Geometry check sheet. Reference: the model listing, model coordinates, mm. A direction names the side the tool comes from. Round coordinates to 2 decimals unless told otherwise and drop trailing zeros. Order: outer loops, then holes, each group sorted by start corner. A loop starts at its lowest first (then second) coordinate and runs counter-clockwise, first axis right, second up. Notation, with made-up numbers: M -23,10.5 L 32,10.5 A28 ccw 32,38.5 Z; hole C 26,-12 d6. An arc over 180 degrees is marked long. Answer as a JSON object with one key per item and string values. Group by question number.
```python
from build123d import *

# Parameters (mm, degrees)
F1_DEPTH = 12.7
F2_R     = 3.175
F3_DEPTH = 3.175
F4_R     = 3.175
F5_DEPTH = 3.175
F6_R     = 3.175
F7_DEPTH = 12.7


with BuildPart() as f1:
    # F0 (on Front) → F1 (new body)
    with BuildSketch(Plane.XZ):
        with BuildLine():
            Line((-8.975765, -6.223), (8.975765, -6.223))
            ThreePointArc((8.975765, -6.223), (0, 10.922), (-8.975765, -6.223))
        make_face()
    extrude(amount=F1_DEPTH)

    # F2 (on face) → F3 (join)
    with BuildSketch(Plane.XZ.offset(12.7)):
        Circle(F2_R)
    extrude(amount=F3_DEPTH)

    # F4 (on face) → F5 (join)
    with BuildSketch(Plane(origin=(0, 0, 0), x_dir=(-1, 0, 0), z_dir=(0, 1, 0))):
        Circle(F4_R)
    extrude(amount=F5_DEPTH)

    # F6 (on face) → F7 (cut)
    with BuildSketch(Plane(origin=(0, 0, -6.223), x_dir=(1, 0, 0), z_dir=(0, 0, -1))):
        with Locations((0, 6.35)):
            Circle(F6_R)
    extrude(amount=-F7_DEPTH, mode=Mode.SUBTRACT)


solid = f1.part
```
1) Sectioned sample at D-D (z = -4). Record the boundary of the cut face in (x, y) (3 decimals), then the cut area to 3 significant figures.
2) Sectioned sample at B-B (x = 0). Record the boundary of the cut face in (y, z) (3 decimals).
3) Sectioned sample at A-A (z = 0). Record the boundary of the cut face in (x, y) (3 decimals), then the cut area to 3 significant figures.
4) Set-up check for faces 1 (the flat face through (0, -6, 6.477)), 2 (the cylindrical face through (0.69, 1.57, -3.1)), 3 (the cylindrical face through (-0.69, -14.27, -3.1)): record each of +Z, -Z, +X, -X, +Y, -Y from which the full face is reachable in a straight line by a thin tool's end or side.
5) Sectioned sample at C-C (y = -6.35). Record the boundary of the cut face in (x, z) (3 decimals), then the cut area to 3 significant figures.
6) Go/stop test with flat-tipped pins: P1, Ø1.5, axis at x = 0, z = 9, coming from the +Y side; P2, Ø8, axis at x = 3, z = 8, coming from the -Y side. Record where each tip stops, or that it passes through.
7) Thickness scan on line 1 along Y through (x, z) = (0, -3) (3 decimals); line 2 along Y through (x, z) = (0, 3.5) (3 decimals); line 3 along X through (y, z) = (-6.35, 0.25) (3 decimals). Record the ranges inside material, lowest first. Write a range as [from, to].
8) Release check for a two-part mould opening along Y. For faces 4 (the flat face through (1.9, -9.1, -6.223)), 5 (the cylindrical face through (1.707, -9.027, 0.038)), 6 (the flat face through (0, 3.175, 0)) record: +Y half, -Y half, draft (parallel to the pull), parting line (faces both ways), or undercut.
Final values:
{
 "1": {"outline": "M -10.163,-12.7 L 10.163,-12.7 L 10.163,0 L -10.163,0 Z; hole C 0,-6.35 d6.35", "area": "226 mm^2"},
 "2": {"outline": "M -15.875,-3.175 L -12.7,-3.175 L -12.7,-6.223 L -9.525,-6.223 L -9.525,6.477 L -3.175,6.477 L -3.175,-6.223 L 0,-6.223 L 0,-3.175 L 3.175,-3.175 L 3.175,3.175 L 0,3.175 L 0,10.922 L -12.7,10.922 L -12.7,3.175 L -15.875,3.175 Z"},
 "3": {"outline": "M -10.922,-12.7 L -3.175,-12.7 L -3.175,-15.875 L 3.175,-15.875 L 3.175,-12.7 L 10.922,-12.7 L 10.922,0 L 3.175,0 L 3.175,3.175 L -3.175,3.175 L -3.175,0 L -10.922,0 Z; hole C 0,-6.35 d6.35", "area": "286 mm^2"},
 "4": {"face 1": "-Z", "face 2": "+Y", "face 3": "-Y"},
 "5": {"outline": "M -8.976,-6.223 L -3.175,-6.223 L -3.175,6.477 L 3.175,6.477 L 3.175,-6.223 L 8.976,-6.223 A10.922 ccw long Z", "area": "235 mm^2"},
 "6": {"P1": "stops at y = 0", "P2": "stops at y = -12.7"},
 "7": {"line 1": "y = [-15.875, -9.525], [-3.175, 3.175]", "line 2": "y = [-12.7, -9.525], [-3.175, 0]", "line 3": "x = [-10.919, -3.175], [3.175, 10.919]"},
 "8": {"face 4": "draft", "face 5": "undercut", "face 6": "+Y half"}
}
